Study the drawing (mm; zero at the part's minimum x, y, z) and answer. Round coordinates to 2 decimals unless told otherwise and drop trailing zeros. Write each loop counter-clockwise with the first axis right and the second up, starting at its lowest first coordinate (ties: lowest second). Pieces come first, ordered by that corner, then holes. Notation, with made-up numbers: (54.5, 15.5) -> (94.5, 15.5) arc R34 ccw to (94.5, 52.5) -> close; hole circle Ø8 at (73, -28). An arc over 180 degrees is marked (long way). Return JSON: item names as keys, results as strings.
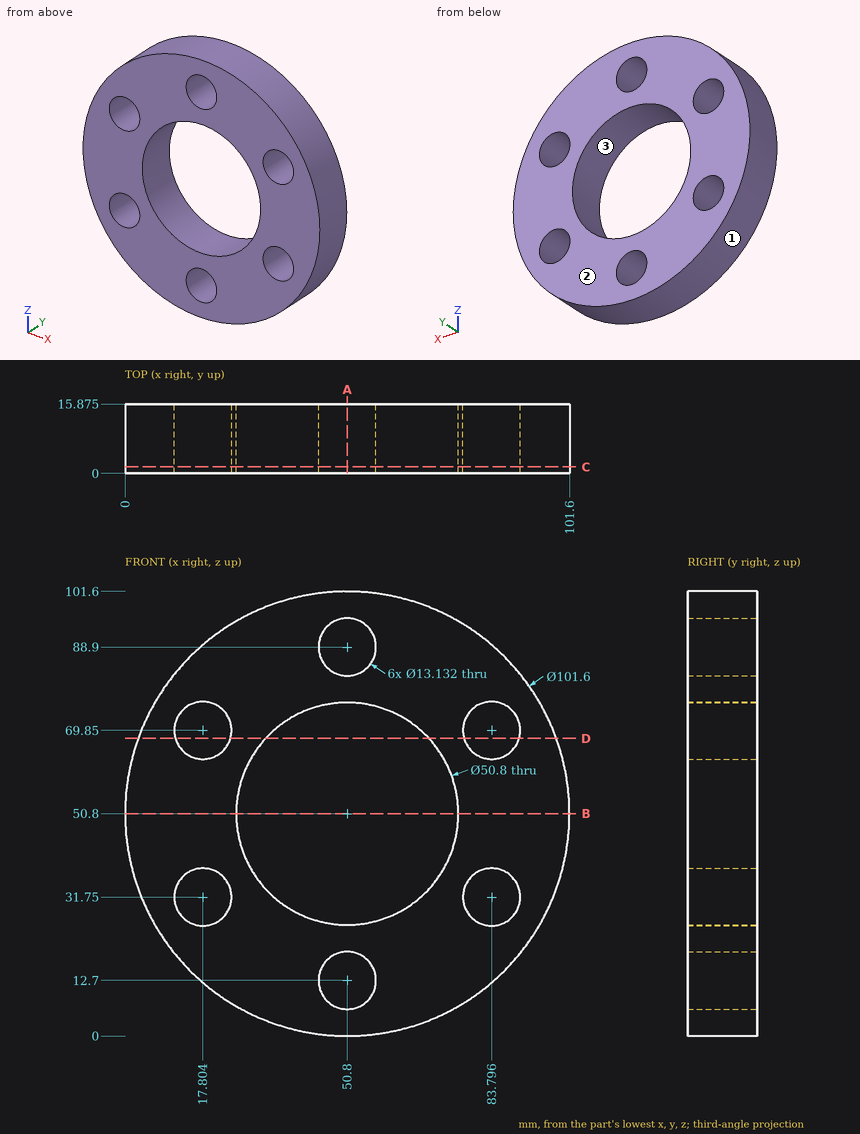
Item 1: Section B-B (z = 50.8) is taken. Give the vertices of the cut face in (x, y) (1 decimal).
Worked answers:
{"outline": "(0, 0) -> (25.4, 0) -> (25.4, 15.9) -> (0, 15.9) -> close; (76.2, 0) -> (101.6, 0) -> (101.6, 15.9) -> (76.2, 15.9) -> close"}
Item 2: Section C-C (y = 1.5) is taken. State how many separate pieces and enclosed holes the cut face has, then the cut area to 3 significant figures.
Worked answers:
{"separate pieces": "1", "enclosed holes": "7", "area": "5,270 mm2"}
Item 3: Flat-ended cylindrical pins translate along their axes: pin 1 (1 mm diameter, centred on x = 80.5, z = 57, fed in from -Y); pin 2 (1.5 mm diameter, centred on x = 27, y = 12, fed in from -Z); pin 3 (10.5 mm diameter, centred on x = 17.8, z = 69.85, fed in from -Y); pin 4 (4 mm diameter, centred on x = 36, y = 6, fed in from +Z). Find the tip coordinate at first contact, or state that the pin passes through.
Worked answers:
{"pin 1": "stops at y = 0", "pin 2": "stops at z = 5.53", "pin 3": "passes through", "pin 4": "stops at z = 99.96"}
Item 4: Section A-A (x = 50.8) is taken. Give the vertices of the cut face in (y, z) (1 decimal).
Worked answers:
{"outline": "(0, 0) -> (15.9, 0) -> (15.9, 6.1) -> (0, 6.1) -> close; (0, 19.3) -> (15.9, 19.3) -> (15.9, 25.4) -> (0, 25.4) -> close; (0, 76.2) -> (15.9, 76.2) -> (15.9, 82.3) -> (0, 82.3) -> close; (0, 95.5) -> (15.9, 95.5) -> (15.9, 101.6) -> (0, 101.6) -> close"}
Item 5: Section D-D (z = 68) is taken. Give the vertices of the cut face in (x, y) (1 decimal).
Worked answers:
{"outline": "(3, 0) -> (11.5, 0) -> (11.5, 15.9) -> (3, 15.9) -> close; (24.1, 0) -> (32.1, 0) -> (32.1, 15.9) -> (24.1, 15.9) -> close; (69.5, 0) -> (77.5, 0) -> (77.5, 15.9) -> (69.5, 15.9) -> close; (90.1, 0) -> (98.6, 0) -> (98.6, 15.9) -> (90.1, 15.9) -> close"}
Item 6: Straight lines are drawn through the part: L1, parallel to Z at x = 50.8, y = 6.75 (1 decimal); L2, parallel to Z at x = 83, y = 6.75; L3, parallel to Z at x = 53, y = 8.5 (1 decimal). For each, find the intervals that lie inside material, in ascending order. Write a range as [from, to].
Worked answers:
{"L1": "z = [0, 6.1], [19.3, 25.4], [76.2, 82.3], [95.5, 101.6]", "L2": "z = [11.51, 25.23], [38.27, 63.33], [76.37, 90.09]", "L3": "z = [0, 6.5], [18.9, 25.5], [76.1, 82.7], [95.1, 101.6]"}
Item 7: For a pull along Z with two mould halves and no side action, classify the marked faces 1, 2 and 3 as released by +Z, released by -Z, zero draft, split by the parting line, or undercut.
Worked answers:
{"face 1": "split by the parting line", "face 2": "zero draft", "face 3": "undercut"}
